Here's the drawing with two shaded views (mm, measured from the low corner). I have some questions. A direction names the side the tool comes from. Round coordinates to 2 decimals unless told otherwise and drop trailing zeros. Loops run counter-clockwise (first coordinate to the right, second up) from the corner with the lowest first, then second, coordinate; pieces in that order, holes last.
(1) Which directions (+Z, -Z, +X, -X, +Y, -Y) give clear straight access to the entire face, cutting with the end or side of a thin tool? Please do the marked faces 1, 2, 3, 4 and 5.
(2) I want a section at D-D on y = 19. Write out the boundary of the cut face in (x, z), plus the area to 4 significant figures.
(3) I want a section at B-B on y = 3.5. Write out the boundary of the cut face in (x, z).
(4) I want a section at A-A on x = 4. Write out the boundary of the cut face in (y, z), plus the area to 3 significant figures.
(5) Thinking about a two-plate mould opening in Y: for the marked faces 6, 7, 8 and 9, which applies, released by +Y, released by -Y, zero draft, split by the parting line, or undercut?
(6) If I drill on line 1 along X through (y, z) = (9, 2.25); line 2 along Y through (x, z) = (38.5, 1.65); line 3 along X through (y, z) = (20.5, 4.6), over which ranges is the centre line in solid material (lowest first)?
(7) Will these pins go through, and if not, where does the flat tip stop? pin 1 Ø0.8 at (x, z) = (5.5, 1.5) entering from -Y; pin 2 Ø2 at (y, z) = (9, 3) entering from +X; pin 3 Ø2.5 at (x, z) = (3.5, 2.5) entering from +Y.
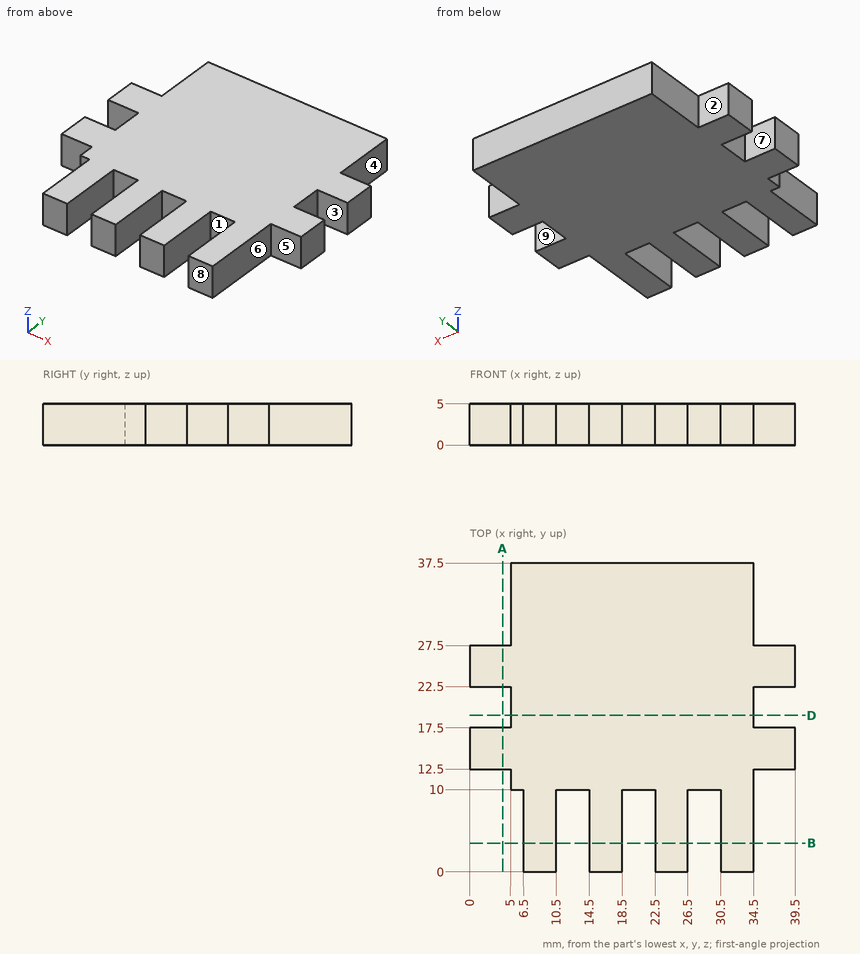
Filled sheet:
1. face 1: +Z, -Z, -Y
1. face 2: +Z, -Z, -X, +Y
1. face 3: +Z, -Z, +X
1. face 4: +Z, -Z, +X, +Y
1. face 5: +Z, -Z, +X, -Y
2. outline: (5, 0) - (34.5, 0) - (34.5, 5) - (5, 5) - close
2. area: 147.5 mm2
3. outline: (6.5, 0) - (10.5, 0) - (10.5, 5) - (6.5, 5) - close; (14.5, 0) - (18.5, 0) - (18.5, 5) - (14.5, 5) - close; (22.5, 0) - (26.5, 0) - (26.5, 5) - (22.5, 5) - close; (30.5, 0) - (34.5, 0) - (34.5, 5) - (30.5, 5) - close
4. outline: (12.5, 0) - (17.5, 0) - (17.5, 5) - (12.5, 5) - close; (22.5, 0) - (27.5, 0) - (27.5, 5) - (22.5, 5) - close
4. area: 50.0 mm2
5. face 6: zero draft
5. face 7: undercut
5. face 8: released by -Y
5. face 9: undercut
6. line 1: x = 6.5 to 10.5, 14.5 to 18.5, 22.5 to 26.5, 30.5 to 34.5
6. line 2: y = 12.5 to 17.5, 22.5 to 27.5
6. line 3: x = 5 to 34.5
7. pin 1: stops at y = 10
7. pin 2: stops at x = 34.5
7. pin 3: stops at y = 27.5
